Can you work these out from the drawing? Everything is in mm from the part's minimum corner. A direction names the side the tool comes from. Coordinates: 2 decimals unless noted, no trailing zeros. Order: outer loops, then holes, each group sorted by start corner. A loop starts at its lowest first (then second) coordinate and runs counter-clockwise, first axis right, second up. Notation, with made-up numbers: (74.5, -4) - (87.5, -4) arc R18 ccw to (87.5, 20) - close; hole circle Ø5 at (1.5, 29.5). An arc over 180 degrees is marked (long way). Use a Markdown table: item, result. Add a question column.
(1) I want a section at B-B (z = 8.5). List the corners of the cut face in (x, y) for me.
(2) For pin 1 Ø9 at (x, z) = (8.5, 8.5) entering from -Y, with a flat end and sliding along its axis, tell me the tip position at first contact or that it passes through.
(3) I want a section at D-D (y = 43). List the corners of the cut face in (x, z) for me.
(4) On a 3-axis mill with a long thin cutter (end or side, diameter ignored), from which of +Z, -Z, +X, -X, +Y, -Y can I reach the whole of each face in a straight line? I mean the marked faces 1 and 2. Say none if no direction works.
(5) I want a section at C-C (x = 7.25). List the corners of the cut face in (y, z) for me, and give its area (3 significant figures).
(6) We'd pull the mould along X, two halves only. Please class the marked faces 3, 4 and 5: pulls with the +X half, pulls with the -X half, needs draft (parallel to the pull), parting line crosses it, or undercut.
(7) I want a section at A-A (y = 30.5). List the corners of the cut face in (x, z) for me, and give its area (3 significant figures).
(8) If I drill on L1, parallel to Z at x = 9.25, y = 30.5; L2, parallel to Y at x = 9.5, z = 11.75; L3, parallel to Z at x = 8.5, y = 18.75, over which ranges is the centre line in solid material (lowest first)? Write a range as [from, to].
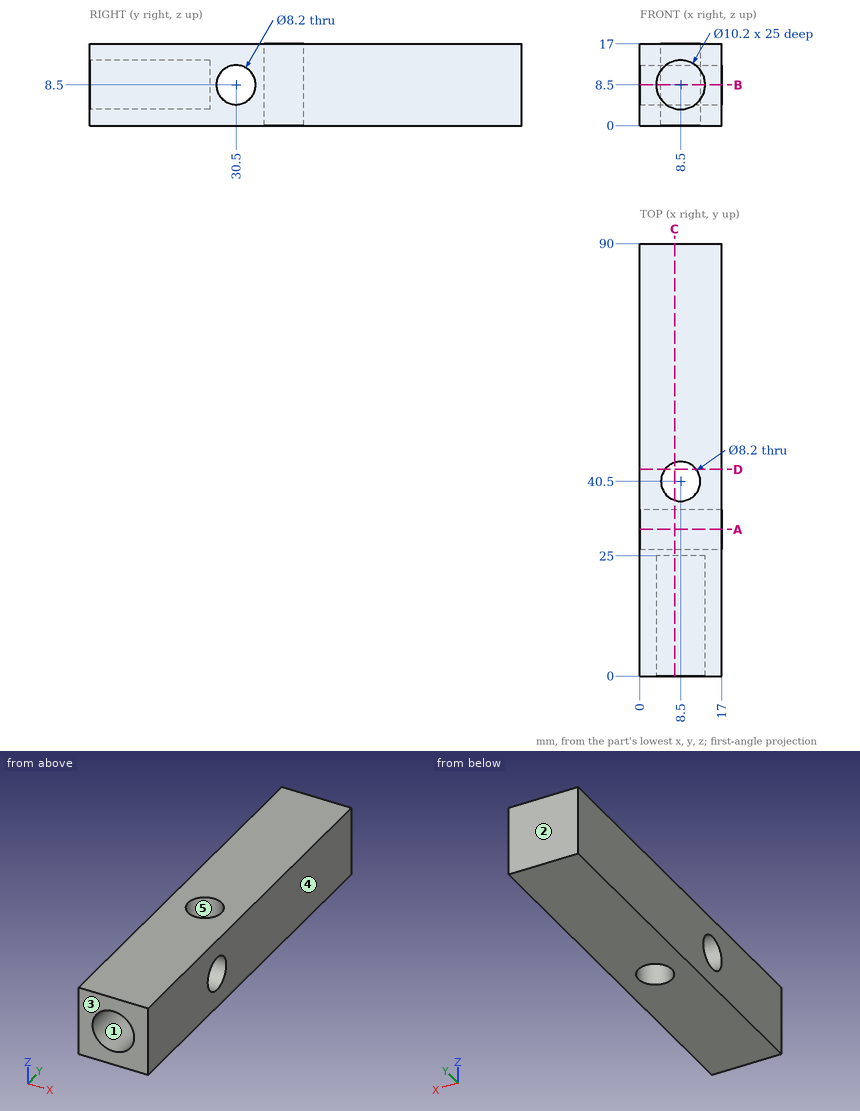
Answers follow:
| question | item | result |
|---|---|---|
| 1 | outline | (0, 0) - (3.4, 0) - (3.4, 25) - (13.6, 25) - (13.6, 0) - (17, 0) - (17, 26.4) - (0, 26.4) - close; (0, 34.6) - (17, 34.6) - (17, 90) - (0, 90) - close; hole circle Ø8.2 at (8.5, 40.5) |
| 2 | pin 1 | stops at y = 25 |
| 3 | outline | (0, 0) - (5.25, 0) - (5.25, 17) - (0, 17) - close; (11.75, 0) - (17, 0) - (17, 17) - (11.75, 17) - close |
| 4 | face 1 | -Y |
| 4 | face 2 | +Z, -Z, +X, -X, +Y |
| 5 | outline | (0, 0) - (36.6, 0) - (36.6, 17) - (0, 17) - (0, 13.44) - (25, 13.44) - (25, 3.56) - (0, 3.56) - close; (44.4, 0) - (90, 0) - (90, 17) - (44.4, 17) - close; hole circle Ø8.2 at (30.5, 8.5) |
| 5 | area | 1,100 mm² |
| 6 | face 3 | needs draft |
| 6 | face 4 | pulls with the +X half |
| 6 | face 5 | undercut |
| 7 | outline | (0, 0) - (17, 0) - (17, 4.4) - (0, 4.4) - close; (0, 12.6) - (17, 12.6) - (17, 17) - (0, 17) - close |
| 7 | area | 150 mm² |
| 8 | L1 | z = [0, 4.4], [12.6, 17] |
| 8 | L2 | y = [25, 28], [33, 36.52], [44.48, 90] |
| 8 | L3 | z = [0, 3.4], [13.6, 17] |
